Geometry check sheet. Reference: the model listing, model coordinates, mm. Round coordinates to 2 decimals unless told otherwise and drop trailing zeros. Order: outer loops, then holes, each group sorted by start corner. A loop starts at its lowest first (then second) coordinate and runs counter-clockwise, first axis right, second up.
(1) Material ranges on line 1 along Z through (x, y) = (-39.5, -0.75); line 2 along Y through (x, z) = (-50, -29), recorded low to high.
(2) Release check for a two-part mould opening along X. For faces 1 (the face through (-53, -2, 0)), 2 (the face through (-75.57, -6.08, 40)), 3 (the face through (75.5, -6.08, -40.07)) record: +X half, -X half, draft (parallel to the pull), parting line (faces both ways), or undercut.
(3) Sectioned sample at D-D (x = -31). Record the boundary of the cut face in (y, z).
(4) Sectioned sample at A-A (z = 4.5). Record the boundary of the cut face in (x, y).
(5) Sectioned sample at B-B (x = -65). Record the boundary of the cut face in (y, z), plus the area to 3 significant figures.
(6) Go/stop test with flat-tipped pins: pin 1 (0.5 mm diameter, centred on y = -12.5, z = 2, fed in from -X); pin 2 (1.5 mm diameter, centred on x = 14, z = -3, fed in from -Y). Record where each tip stops, or that it passes through.
(7) Sectioned sample at C-C (z = 16). Record the boundary of the cut face in (x, y).
from build123d import *

# Parameters (mm, degrees)
F0_W     = 154
F0_H     = 83
F1_DEPTH = 12
F2_R     = 5
F3_W     = 6.5
F3_H     = 17.5
F4_DEPTH = 1
F5_R     = 2.5
F6_W     = 28
F6_H     = 19
F7_DEPTH = 2


with BuildPart() as f1:
    # F0 (on Front) → F1 (new body)
    with BuildSketch(Plane.XZ):
        Rectangle(F0_W, F0_H)
    extrude(amount=F1_DEPTH)

    # F2
    f2_edges = [f1.edges().sort_by_distance(p)[0] for p in [
        (-77, -6, 41.5),
        (77, -6, 41.5),
        (77, -6, -41.5),
        (-77, -6, -41.5),
    ]]
    fillet(f2_edges, radius=F2_R)

    # F3 (on face) → F4 (join)
    with BuildSketch(Plane.XZ.offset(12)):
        with Locations((67.75, 0)):
            Rectangle(F3_W, F3_H)
    extrude(amount=F4_DEPTH)

    # F5
    f5_edges = [f1.edges().sort_by_distance(p)[0] for p in [
        (71, -12.5, -8.75),
        (71, -12.5, 8.75),
        (64.5, -12.5, 8.75),
        (64.5, -12.5, -8.75),
    ]]
    fillet(f5_edges, radius=F5_R)

    # F6 (on Front) → F7 (cut)
    with BuildSketch(Plane.XZ):
        with Locations((-53, 0)):
            Rectangle(F6_W, F6_H)
    extrude(amount=F7_DEPTH, mode=Mode.SUBTRACT)


solid = f1.part
Answer below:
1. line 1: z = -41.5 to -9.5, 9.5 to 41.5
1. line 2: y = -12 to 0
2. face 1: undercut
2. face 2: -X half
2. face 3: +X half
3. outline: (-12, -41.5) - (0, -41.5) - (0, 41.5) - (-12, 41.5) - close
4. outline: (-77, -12) - (64.5, -12) - (64.5, -13) - (71, -13) - (71, -12) - (77, -12) - (77, 0) - (-39, 0) - (-39, -2) - (-67, -2) - (-67, 0) - (-77, 0) - close
5. outline: (-12, -41.5) - (0, -41.5) - (0, -9.5) - (-2, -9.5) - (-2, 9.5) - (0, 9.5) - (0, 41.5) - (-12, 41.5) - close
5. area: 958 mm2
6. pin 1: stops at x = 64.5
6. pin 2: stops at y = -12
7. outline: (-77, -12) - (77, -12) - (77, 0) - (-77, 0) - close
